CAD build for the part. Positions are in the model's coordinates, mm. Coordinates: 2 decimals unless noted, no trailing zeros. Loops run counter-clockwise (first coordinate to the right, second up) from the corner with the lowest first, then second, coordinate; pieces in that order, holes last. Notation, with made-up numbers: (13.25, 77) -> (20.25, 77) arc R19 cw to (20.25, 114) -> close; hole circle Ø9 at (34.25, -23.75). An arc over 180 degrees is marked (long way). Write item = value, one per line. Start each with the question number.
(1) Band-saw the part on D-D (x = -51.75). Write the cut outline in (y, z).
(2) Flat gauge pins, fed straight in: P1, Ø3, axis at x = -52.5, y = 51.5, coming from the +Z side; P2, Ø3.5, axis at x = -55, z = -51, coming from the -Y side. Where does each tip first touch, or does it go through?
(3) Band-saw the part on B-B (x = -55). Write the cut outline in (y, z).
(4) Band-saw the part on A-A (z = -51). Write the cut outline in (x, y).
(5) Band-saw the part on C-C (y = 10). Write the cut outline in (x, z), and give its area (3 significant figures).
(6) Drill centre lines: line 1 (X direction, y = 37, z = -51.25); line 2 (Z direction, x = -55, y = 39); line 3 (X direction, y = 28, z = -51.5). Where is each one in solid material? Low to high. Write a range as from..to.
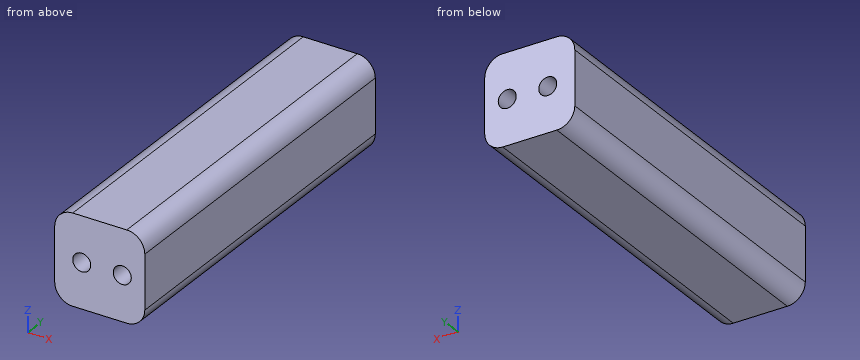
```python
from build123d import *

# Parameters (mm, degrees)
CYLINDER050_R       = 2
CYLINDER050_DEPTH   = 100
ARRAY001028_X_COUNT = 2
ARRAY001028_X_PITCH = 9
BOX028_W            = 20
BOX028_H            = 80
BOX028_DEPTH        = 20
FILLET_R            = 4


with BuildPart() as stand_attachment_hole_fusion001:
    # Cylinder050 → Cylinder050 (new body)
    with BuildSketch(Plane(origin=(0, -10, 10), x_dir=(1, 0, 0), z_dir=(0, 1, 0))):
        Circle(CYLINDER050_R)
    extrude(amount=CYLINDER050_DEPTH)

    # Array001028 X: stand attachment hole fusion001 ×2


with BuildPart() as stand_attachment_hole_fusion001_1:
    add(stand_attachment_hole_fusion001.part)
    with Locations(*[(i * ARRAY001028_X_PITCH, 0, 0) for i in range(1, ARRAY001028_X_COUNT)]):
        add(stand_attachment_hole_fusion001.part)


with BuildPart() as stand_attachment_middle_fillet:
    # Box028 → Box028 (new body)
    with BuildSketch(Plane(origin=(-6, 0, 0), x_dir=(1, 0, 0), z_dir=(0, 0, 1))):
        with Locations((10, 40)):
            Rectangle(BOX028_W, BOX028_H)
    extrude(amount=BOX028_DEPTH)

    # Cut020: cut stand attachment hole fusion001
    add(stand_attachment_hole_fusion001_1.part, mode=Mode.SUBTRACT)


with BuildPart() as stand_attachment_middle_fillet_1:
    # Cut020 placement: moved
    add(stand_attachment_middle_fillet.part.moved(Location((-64, 0, -61))))

    # Fillet
    fillet_edges = [stand_attachment_middle_fillet_1.edges().sort_by_distance(p)[0] for p in [
        (-70, 40, -41),
        (-70, 40, -61),
        (-50, 40, -41),
        (-50, 40, -61),
    ]]
    fillet(fillet_edges, radius=FILLET_R)


solid = stand_attachment_middle_fillet_1.part
```
Findings below:
q1.outline = (0, -60.31) -> (80, -60.31) -> (80, -41.69) -> (0, -41.69) -> close
q2.P1 = -41
q2.P2 = through
q3.outline = (0, -61) -> (80, -61) -> (80, -53) -> (0, -53) -> close; (0, -49) -> (80, -49) -> (80, -41) -> (0, -41) -> close
q4.outline = (-70, 0) -> (-66, 0) -> (-66, 80) -> (-70, 80) -> close; (-62, 0) -> (-57, 0) -> (-57, 80) -> (-62, 80) -> close; (-53, 0) -> (-50, 0) -> (-50, 80) -> (-53, 80) -> close
q5.outline = (-70, -57) arc R4 ccw to (-66, -61) -> (-54, -61) arc R4 ccw to (-50, -57) -> (-50, -45) arc R4 ccw to (-54, -41) -> (-66, -41) arc R4 ccw to (-70, -45) -> close; hole circle Ø4 at (-64, -51); hole circle Ø4 at (-55, -51)
q5.area = 361 mm²
q6.line_1 = -70..-65.98, -62.02..-56.98, -53.02..-50
q6.line_2 = -61..-53, -49..-41
q6.line_3 = -70..-65.94, -62.06..-56.94, -53.06..-50
